Design review of the part shown in the three views and the two pictorial views. Dimensions are in mm from the part's minimum x, y and z. Coordinates: 2 decimals unless noted, no trailing zeros. Loops run counter-clockwise (first coordinate to the right, second up) from the corner with the lowest first, then second, coordinate; pieces in that order, holes last. Notation, with made-up numbers: (45.5, 58.5) -> (85.5, 58.5) arc R12 cw to (85.5, 74.5) -> close; hole circle Ø9 at (47, -19). An arc over 180 degrees is marked (long way). One line per item, written item: value.
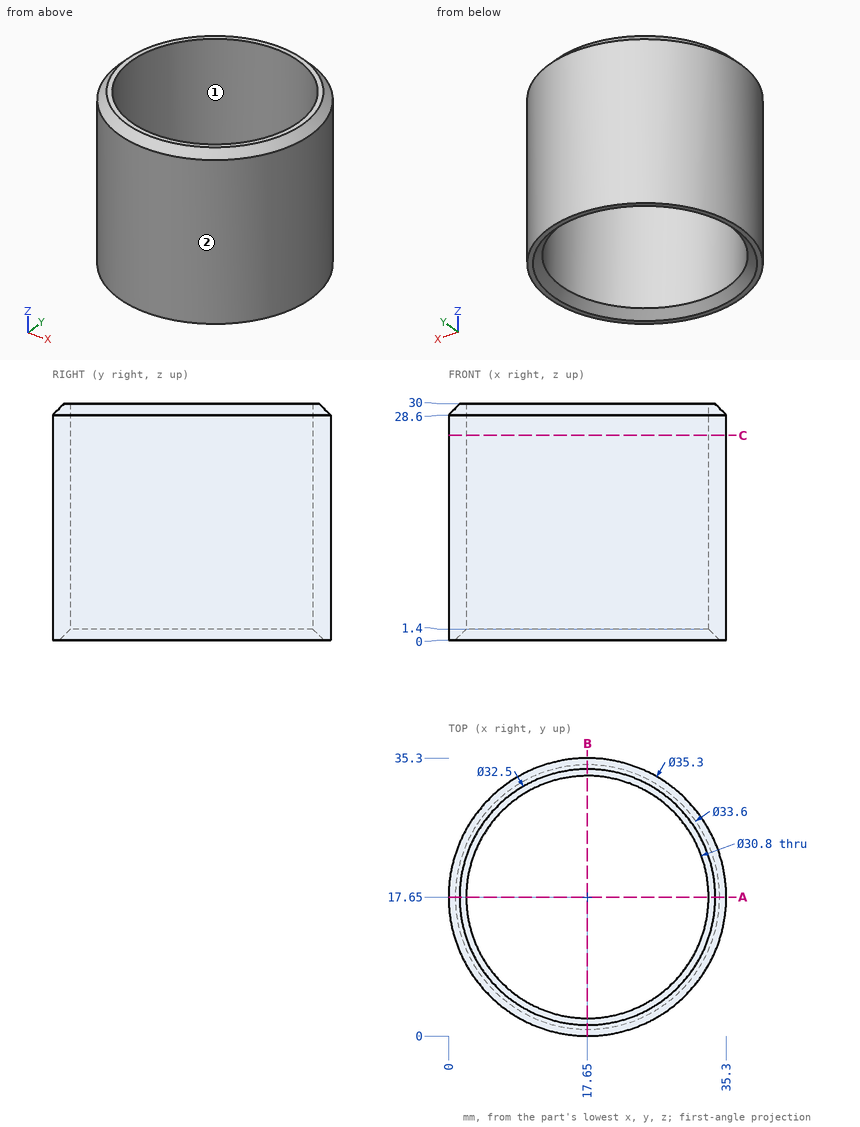
1. Take a section at A-A, the plane y = 17.65. Give the boundary of the cut face in (x, z), and give its area (3 significant figures).
Return value:
outline: (0, 0) -> (0.85, 0) -> (2.25, 1.4) -> (2.25, 30) -> (1.4, 30) -> (0, 28.6) -> close; (33.05, 1.4) -> (34.45, 0) -> (35.3, 0) -> (35.3, 28.6) -> (33.9, 30) -> (33.05, 30) -> close
area: 131 mm2
2. Take a section at C-C, the plane z = 26. Give the boundary of the cut face in (x, y).
Return value:
outline: circle Ø35.3 at (17.65, 17.65); hole circle Ø30.8 at (17.65, 17.65)
3. Insertion check: pin 1 Ø12 at (x, z) = (25.5, 16.5) entering from -Y; pin 2 Ø12 at (y, z) = (13.5, 20) entering from +X; pin 3 Ø8 at (y, z) = (6, 17) entering from +X; pin 4 Ø1.5 at (x, y) = (8.5, 5) entering from -Z. Each pin has a flat end and moves straight along its axis. Give the tip position at first contact, or say it passes through.
Return value:
pin 1: stops at y = 0.1
pin 2: stops at x = 35.3
pin 3: stops at x = 33.56
pin 4: stops at z = 0.44
4. The part is to be moulded in two halves that separate along Y. For the marked faces 1 and 2, say which applies: pulls with the +Y half, pulls with the -Y half, needs draft (parallel to the pull), parting line crosses it, or undercut.
Return value:
face 1: undercut
face 2: parting line crosses it
5. To check wall thickness, follow probe 1 along Y at (x, z) = (17.65, 20.5); probe 2 along X at (y, z) = (11.5, 25.5); probe 3 along Y at (x, z) = (23, 21). State the ranges of each line that lie inside material, in increasing order. Write a range as from..to.
Return value:
probe 1: y = 0..2.25, 33.05..35.3
probe 2: x = 1.11..3.53, 31.77..34.19
probe 3: y = 0.83..3.21, 32.09..34.47
